Autodesk Inventor part; units mm, degrees
ref_plane "YZ Plane" through (0, 0, 0) normal (1, 0, 0) x (0, 1, 0)
ref_plane "XZ Plane" through (0, 0, 0) normal (0, 1, 0) x (-1, 0, 0)
ref_plane "XY Plane" through (0, 0, 0) normal (0, 0, 1) x (1, 0, 0)
sketch "Sketch1" plane through (0, 0, 0) normal (0, 0, 1) x (1, 0, 0)
  line L0 (0, 0) -> (21.9, 0)
  line L1 (21.9, 0) -> (21.9, 25)
  line L2 (21.9, 25) -> (0, 25)
  line L3 (0, 25) -> (0, 0)
  line L4 (21.9, 25) -> (2, 25)
  line L5 (2, 25) -> (2, 2)
  line L6 (2, 2) -> (21.9, 2)
  line L7 (21.9, 2) -> (21.9, 25)
  point P0 (21.9, 2)
  dimension "d0" = 21.9
  dimension "d1" = 25
  dimension "d2" = 2
  dimension "d3" = 2
extrude "Extrusion1" add sketch "Sketch1" against normal blind 20 contours L3 L2 L5 L6 L1 L0
sketch "Sketch2" plane through (0, 0, 0) normal (-1, 0, 0) x (0, 0, 1)
  line L0 (-20, 2) -> (-20, 0)
  line L1 (-20, 0) -> (-20, 18.8)
  line L2 (-20, 18.8) -> (0, 18.8)
  line L3 (0, 25) -> (0, 0)
  circle A0 centre (-14.75, 18.8) radius 1.5
  circle A1 centre (-5.25, 18.8) radius 1.5
  dimension "d6" = 18.8
  dimension "d7" = 3
  dimension "d8" = 3
  dimension "d9" = 9.5
  dimension "d10" = 5.25
extrude "Extrusion2" cut sketch "Sketch2" against normal through all
sketch "Sketch4" plane through (2, 2, 0) normal (0, 1, 0) x (1, 0, 0)
  line L0 (0, 0) -> (0, 20)
  line L1 (0, 10) -> (13.5, 10)
  circle A0 centre (13.5, 10) radius 2.6
  point P0 (-2, 0)
  dimension "d13" = 13.5
  dimension "d14" = 5.2
extrude "Extrusion3" cut sketch "Sketch4" against normal through all
properties part number "LimitSwitch Center Gantry Mount"
Input: part model. Units: mm. Frame: model coordinates. A direction names the side the tool comes from. Give positions to 0.01 mm unless a question says otherwise; leave off trailing zeros. Write each loop counter-clockwise with the first axis right and the second up, starting at its lowest first coordinate (ties: lowest second). Pieces come first, ordered by that corner, then holes. Notation, with made-up numbers: (18, -1.75) -> (46, -1.75) arc R13 cw to (46, 23.25) -> close; hole circle Ø5 at (89.25, 0.5). An arc over 180 degrees is marked (long way). Use one line per item in the form item = value. Start each with the question number.
1) Section query A-A on z = -10. Return the cut outline in (x, y), then the cut area to 3 significant figures.
2) Draft query along Z for faces 1 (the flat face through (1, 8, 0)), 2 (the cylindrical face through (17.9, 1, -9)), 3 (the flat face through (11, 0, -10)), 4 (the cylindrical face through (0.986, 17.336, -15.075)). Return one class per face: pulls with the +Z half, pulls with the -Z half, needs draft (parallel to the pull), parting line crosses it, or undercut.
3) Pin query (flat end, axial travel): pin 1 (4 mm diameter, centred on x = 10.5, z = -12.5, fed in from +Y); pin 2 (2 mm diameter, centred on y = 21, z = -10, fed in from +X). Return the tip coordinate at first contact, or that it passes through.
4) Section query B-B on y = 18.8. Return the cut outline in (x, z).
5) Section query C-C on x = 16.5. Return the cut outline in (y, z).
6) Ray query, probe 1 along Y at (x, z) = (1.35, -5.25); probe 2 along X at (y, z) = (1.55, -10); probe 3 along Z at (x, y) = (15.5, 1.6). Return the intervals inside material, ascending. Write a range as from..to.
7) Set-up query: faces 5 (the flat face through (2, 14, -10)), 6 (the cylindrical face through (0.986, 17.336, -5.575)). Return all of +Z, -Z, +X, -X, +Y, -Y with unobstructed straight access to the full face (end or side cutting, diameter ignored); none if empty.
8) Section query D-D on z = -5.25. Return the cut outline in (x, y), then the cut area to 3 significant figures.
Outcome:
q1.outline = (0, 0) -> (12.9, 0) -> (12.9, 2) -> (2, 2) -> (2, 25) -> (0, 25) -> close; (18.1, 0) -> (21.9, 0) -> (21.9, 2) -> (18.1, 2) -> close
q1.area = 79.4 mm^2
q2.face_1 = pulls with the +Z half
q2.face_2 = undercut
q2.face_3 = needs draft
q2.face_4 = undercut
q3.pin_1 = 2
q3.pin_2 = 2
q4.outline = (0, -20) -> (2, -20) -> (2, -16.25) -> (0, -16.25) -> close; (0, -13.25) -> (2, -13.25) -> (2, -6.75) -> (0, -6.75) -> close; (0, -3.75) -> (2, -3.75) -> (2, 0) -> (0, 0) -> close
q5.outline = (0, -20) -> (2, -20) -> (2, -12.4) -> (0, -12.4) -> close; (0, -7.6) -> (2, -7.6) -> (2, 0) -> (0, 0) -> close
q6.probe_1 = 0..17.3, 20.3..25
q6.probe_2 = 0..12.9, 18.1..21.9
q6.probe_3 = -20..-12.6, -7.4..0
q7.face_5 = +Z, -Z, +X, +Y
q7.face_6 = +X, -X
q8.outline = (0, 0) -> (21.9, 0) -> (21.9, 2) -> (2, 2) -> (2, 17.3) -> (0, 17.3) -> close; (0, 20.3) -> (2, 20.3) -> (2, 25) -> (0, 25) -> close
q8.area = 83.8 mm^2
